Autodesk Inventor part; units mm, degrees
ref_plane "YZ Plane" through (0, 0, 0) normal (1, 0, 0) x (0, 1, 0)
ref_plane "XZ Plane" through (0, 0, 0) normal (0, 1, 0) x (-1, 0, 0)
ref_plane "XY Plane" through (0, 0, 0) normal (0, 0, 1) x (1, 0, 0)
sketch "스케치1" plane through (0, 0, 0) normal (0, 0, 1) x (1, 0, 0)
  circle A0 centre (0, 0) radius 14
  line L0 (-7.25, -10.8235) -> (7.25, -10.8235) construction
  line L1 (7.25, -10.8235) -> (7.25, -17.1765)
  line L2 (7.25, -17.1765) -> (-7.25, -17.1765)
  line L3 (-7.25, -17.1765) -> (-7.25, -10.8235)
  line L4 (-7.25, -10.8235) -> (7.25, -17.1765) construction
  line L5 (7.25, -10.8235) -> (-7.25, -17.1765) construction
  line L6 (7.25, -11.9765) -> (7.25, -17.1765)
  line L7 (0, -14) -> (0, 0)
  point P0 (-7.25, -11.9765)
  dimension "d0" = 28
  dimension "d1" = 5.2
  dimension "d2" = 14.5
extrude "돌출1" add sketch "스케치1" against normal blind 19.2 contours A0
extrude "돌출2" add sketch "스케치1" against normal blind 16.6 contours A0 L1 L2 L3
sketch "스케치2" plane through (0, 0, 0) normal (0, 0, 1) x (1, 0, 0)
  circle A0 centre (-17.6, 0) radius 2.1
  circle A1 centre (-17.6, 0) radius 3.5
  line L0 (-17.6, 3.5) -> (-13.5554, 3.5)
  line L1 (-17.6, -3.5) -> (-13.5554, -3.5)
  line L2 (-17.6, 0) -> (0, 0)
  arc A2 (7.25, -11.9765) -> (-7.25, -11.9765) centre (0, 0) ccw
  dimension "d7" = 4.2
  dimension "d8" = 7
  dimension "d9" = 17.6
extrude "돌출3" add sketch "스케치2" against normal blind 1
mirror "미러1" about plane through (0, 0, 0) normal (1, 0, 0) of "돌출3"
sketch "스케치3" plane through (0, 0, 0) normal (0, 0, 1) x (1, 0, 0)
  circle A0 centre (0, 7.8) radius 4.6
  line L0 (0, 12.4) -> (0, 14)
  arc A1 (13.5554, 3.5) -> (-13.5554, 3.5) centre (0, 0) ccw
  line L1 (0, 7.8) -> (0, 0)
  point P0 (0, 14)
  dimension "d12" = 9.2
  dimension "d13" = 1.6
extrude "돌출4" add sketch "스케치3" along normal blind 1.5
sketch "스케치4" plane through (0, 7.8, 1.5) normal (0, 0, 1) x (1, 0, 0)
  circle A0 centre (0, 0) radius 4.6
  circle A1 centre (0, 0) radius 2.5
  point P0 (0, -7.8)
  dimension "d16" = 5
extrude "돌출5" add sketch "스케치4" along normal blind 8 contours A1
sketch "스케치5" plane through (0, 7.8, 9.5) normal (0, 0, 1) x (1, 0, 0)
  circle A0 centre (0, 0) radius 2.5
  line L0 (-2.5, 1.5) -> (2.5, 1.5)
  line L1 (2.5, 1.5) -> (2.5, -1.5)
  line L2 (2.5, -1.5) -> (-2.5, -1.5)
  line L3 (-2.5, -1.5) -> (-2.5, 1.5)
  line L4 (-2.5, 1.5) -> (2.5, -1.5) construction
  line L5 (2.5, 1.5) -> (-2.5, -1.5) construction
  point P0 (0, -7.8)
  point P1 (2, -1.5)
  point P2 (-2, -1.5)
  point P3 (-2, 1.5)
  point P4 (2, 1.5)
  dimension "d19" = 3
extrude "돌출6" cut sketch "스케치5" against normal blind 6 contours L0 A0 | A0 L2
ref_plane "작업 평면1" through (0, 0, 0) normal (1, 0, 0) x (0, 1, 0)
properties part number "스텝모터"
Source: CAD feature listing. Evaluate the final solid. Frame: model axes, mm. A direction names the side the tool comes from. Give positions to 0.01 mm unless a question says otherwise; leave off trailing zeros. Write each loop counter-clockwise with the first axis right and the second up, starting at its lowest first coordinate (ties: lowest second). Pieces come first, ordered by that corner, then holes.
1. First-contact query: pin 1 (0.5 mm diameter, centred on x = 0.5, y = 6, fed in from +Z); pin 2 (1.5 mm diameter, centred on y = -7, z = 2, fed in from +X) (3 decimals); pin 3 (1.5 mm diameter, centred on y = 2, z = -10, fed in from -X); pin 4 (0.5 mm diameter, centred on x = 16.5, z = -0.5, fed in from +Y). Flat tips, straight axial feed; report the tip coordinate or a pass-through.
2. Access query for faces 1 (the face through (0, 9.3, 7)), 2 (the face through (7.25, -15, -8)), 3 (the face through (15.5, 3.5, -0.5)). Directions: +Z, -Z, +X, -X, +Y, -Y. A direction counts if a zero-diameter tool reaches every point of the face in a straight line with its end or side. Return the directions, or none.
3. Section query B-B (x = 16.5). Return the cut outline in (y, z), then the cut area to 3 significant figures.
4. Section query C-C (y = -13). Return the cut outline in (x, z), then the cut area to 3 significant figures.
5. Section query A-A (x = 0). Return the cut outline in (y, z), then the cut area to 3 significant figures.
6. Section query D-D (z = 1). Return the cut outline in (x, y), then the cut area to 3 significant figures.
7. Material intervals for line 1 along Y through (x, z) = (17.6, -0.75); line 2 along Z through (x, y) = (-0.5, 5); line 3 along Z through (x, y) = (-15, 2), sorted ascending.
Output values:
1. pin 1: stops at z = 3.5
1. pin 2: passes through
1. pin 3: stops at x = -13.94
1. pin 4: stops at y = 3.5
2. face 1: +Z, +X, -X, +Y
2. face 2: +Z, -Z, +X, -Y
2. face 3: +Z, -Z, +X, +Y
3. outline: (-3.5, -1) - (-1.79, -1) - (-1.79, 0) - (-3.5, 0) - close; (1.79, -1) - (3.5, -1) - (3.5, 0) - (1.79, 0) - close
3. area: 3.42 mm2
4. outline: (-7.25, -16.6) - (-5.2, -16.6) - (-5.2, -19.2) - (5.2, -19.2) - (5.2, -16.6) - (7.25, -16.6) - (7.25, 0) - (-7.25, 0) - close
4. area: 268 mm2
5. outline: (-17.18, -16.6) - (-14, -16.6) - (-14, -19.2) - (14, -19.2) - (14, 0) - (12.4, 0) - (12.4, 1.5) - (10.3, 1.5) - (10.3, 3.5) - (9.3, 3.5) - (9.3, 9.5) - (6.3, 9.5) - (6.3, 3.5) - (5.3, 3.5) - (5.3, 1.5) - (3.2, 1.5) - (3.2, 0) - (-17.18, 0) - close
5. area: 632 mm2
6. outline: circle Ø9.2 at (0, 7.8)
6. area: 66.5 mm2
7. line 1: y = -3.5 to -2.1, 2.1 to 3.5
7. line 2: z = -19.2 to 1.5
7. line 3: z = -1 to 0
